from build123d import *

# Parameters (mm, degrees)
SKETCH1_R           = 37
BOSS_EXTRUDE1_DEPTH = 30.05
SKETCH2_R           = 3.175
BOSS_EXTRUDE2_DEPTH = 0.6
SKETCH3_R           = 0.375
BOSS_EXTRUDE3_DEPTH = 12
FILLET1_R           = 2


with BuildPart() as part:
    # Sketch1 → Boss-Extrude1 (new body)
    with BuildSketch(Plane.XY):
        Circle(SKETCH1_R)
    extrude(amount=-BOSS_EXTRUDE1_DEPTH)

    # Sketch2 → Boss-Extrude2 (add)
    with BuildSketch(Plane.XY):
        Circle(SKETCH2_R)
    extrude(amount=BOSS_EXTRUDE2_DEPTH)

    # Sketch3 → Boss-Extrude3 (add)
    with BuildSketch(Plane.XY.offset(0.6)):
        Circle(SKETCH3_R)
    extrude(amount=BOSS_EXTRUDE3_DEPTH)

    # Fillet1
    fillet1_edges = [part.edges().sort_by_distance(p)[0] for p in [
        (-37, 0, 0),
        (-37, 0, -30.05),
    ]]
    fillet(fillet1_edges, radius=FILLET1_R)


solid = part.part
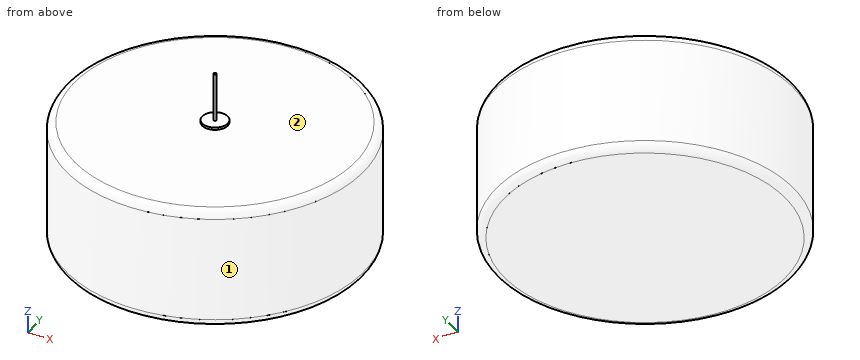
Input: part model. Units: mm. Frame: model coordinates. Face numbers are marked on the shaded views. Round coordinates to 2 decimals unless told otherwise and drop trailing zeros. Loops run counter-clockwise (first coordinate to the right, second up) from the corner with the lowest first, then second, coordinate; pieces in that order, holes last. Notation, with made-up numbers: M 44.25,-18.75 L 94.25,-18.75 A27 ccw 94.25,13.25 Z; hole C -10.5,-12 d5. An arc over 180 degrees is marked long. Answer as CSV lines item,"result". Start each with the question number.
(1) Draft query along Y for the marked faces 1 and 2. Return one class per face: released by +Y, released by -Y, zero draft, split by the parting line, or undercut.
(2) Line query: line 1 (Z direction, x = 2.5, y = -28); line 2 (Y direction, x = -1, z = -4); line 3 (X direction, y = -12.5, z = -1). Output: solid intervals per line, ascending. Write a range as [from, to].
(3) Section A-A, the plane z = -18. Output: boundary loops of the cut face in (x, y).
(4) First-contact query: pin 1 (6 mm diameter, centred on y = -11, z = -8.5, fed in from +X); pin 2 (8 mm diameter, centred on x = 9, y = -29, fed in from +Z); pin 3 (1.9 mm diameter, centred on x = -1.5, y = -0.5, fed in from +Z). Flat tips, straight axial feed; report the tip coordinate or a pass-through.
(5) Section B-B, the plane z = 10. Output: boundary loops of the cut face in (x, y) (3 decimals), plus the area to 3 significant figures.
Values found:
1,face 1,"split by the parting line"
1,face 2,"zero draft"
2,line 1,"z = [-30.05, 0]"
2,line 2,"y = [-36.99, 36.99]"
2,line 3,"x = [-34.54, 34.54]"
3,outline,"C 0,0 d74"
4,pin 1,"stops at x = 36.12"
4,pin 2,"stops at z = 0"
4,pin 3,"stops at z = 0.6"
5,outline,"C 0,0 d0.75"
5,area,"0.442 mm²"
